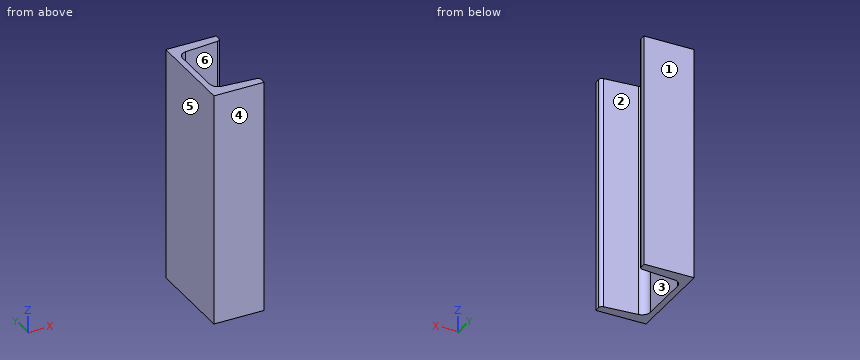
Autodesk Inventor part; units mm, degrees
ref_plane "Начальная плоскость" through (0, 0, 0) normal (0, 0, 1) x (1, 0, 0)
ref_plane "Конечная плоскость" through (0, 0, 168) normal (0, 0, 1) x (1, 0, 0)
ref_plane "YZ Plane" through (0, 0, 0) normal (1, 0, 0) x (0, 1, 0)
ref_plane "Начальная плоскость" through (0, 0, 0) normal (0, 0, 1) x (1, 0, 0)
ref_plane "Конечная плоскость" through (0, 0, 168) normal (0, 0, 1) x (1, 0, 0)
sketch "Эскиз" plane through (0, 0, 0) normal (0, 0, 1) x (1, 0, 0)
  line L0 (36, -32.5) -> (0, -32.5)
  line L1 (36, -32.5) -> (36, -28.696)
  line L2 (33.6994, -26.2039) -> (9.9215, -24.3017)
  line L3 (4.4, -18.3208) -> (4.4, 18.3208)
  line L4 (33.6994, 26.2039) -> (9.9215, 24.3017)
  line L5 (36, 28.696) -> (36, 32.5)
  line L6 (0, 32.5) -> (36, 32.5)
  line L7 (0, -32.5) -> (0, 32.5)
  arc A0 (4.4, -18.3208) -> (9.9215, -24.3017) centre (10.4, -18.3208) ccw
  arc A1 (9.9215, 24.3017) -> (4.4, 18.3208) centre (10.4, 18.3208) ccw
  arc A2 (36, -28.696) -> (33.6994, -26.2039) centre (33.5, -28.696) ccw
  arc A3 (33.6994, 26.2039) -> (36, 28.696) centre (33.5, 28.696) ccw
  line L8 (0, 45.5) -> (0, -45.5) construction
  line L9 (-7.2974, 0) -> (43.7847, 0) construction
  point P0 (36, -26.388)
  point P1 (4.4, -23.86)
  point P2 (4.4, 23.86)
  point P3 (36, 26.388)
  dimension "d3" = 36
  dimension "d5" = 4.4
  dimension "d7" = 65
  dimension "d9" = 8.64
  dimension "d11" = 8.64
  dimension "d13" = 6.112
  dimension "d15" = 6.112
  dimension "d22" = 6
  dimension "d23" = 2.5
  dimension "d24" = 32.5
  dimension "d25" = 0
extrude "Тело" add sketch "Эскиз" along normal up to surface (168 mm away) from surface at 0
sketch "Sketch3" plane through (0, 0, 0) normal (0, 0, 1) x (1, 0, 0)
  line L0 (0, 0) -> (10, 0)
ref_plane "Work Plane7" through (0, 0, 0) normal (0, -1, 0) x (1, 0, 0)
sketch "Sketch4" plane through (0, 0, 0) normal (0, -1, 0) x (1, 0, 0)
  line L0 (-2, 0) -> (12, 0)
  line L1 (-2, 168) -> (12, 168)
  dimension "d29" = 168
equation "\"d3\" = b"
equation "\"d7\" = ParH"
equation "\"d22\" = R"
equation "\"d23\" = R1"
equation "\"d24\" = 0.5 * d7"
equation "\"d16\" = G_L"
equation "\"R1\" = 2.5"
equation "\"R\" = 6"
equation "\"t1\" = 4.4"
equation "\"t2\" = 7.2"
equation "\"ParH\" = 65"
equation "\"b\" = 36"
equation "\"msp_x1\" = 0.04 * b"
equation "\"msp_x2\" = -0.08 * t1 + 0.04 * b"
equation "\"G_L\" = d29"
equation "\"ex\" = 0"
equation "\"G_OFFSET_START\" = 0"
equation "\"G_OFFSET_END\" = 0"
equation "\"d27\" = G_OFFSET_END + B_L"
equation "\"B_L\" = 168"
properties part number "Швеллер 6.5U-168 ГОСТ 8240-97" material "Сталь, мягкая"
Build history of the part. All positions in model axes, mm. Face numbers are marked on the shaded views. A direction names the side the tool comes from. Round coordinates to 2 decimals unless told otherwise and drop trailing zeros. Order: outer loops, then holes, each group sorted by start corner. A loop starts at its lowest first (then second) coordinate and runs counter-clockwise, first axis right, second up. Notation, with made-up numbers: (72.5, -10.75) - (98.5, -10.75) arc R15 ccw to (98.5, 10.25) - close; hole circle Ø5 at (-20, 10). An arc over 180 degrees is marked (long way). Use a Markdown table: item, result.
1) Pull direction Y, two halves, no side cores. Call the marked faces 3, 4, 5 and 6: pulls with the +Y half, pulls with the -Y half, needs draft (parallel to the pull), parting line crosses it, or undercut.
Recorded:
| item | result |
|---|---|
| face 3 | undercut |
| face 4 | pulls with the -Y half |
| face 5 | needs draft |
| face 6 | undercut |
2) Saw through at C-C on y = 2.5. Write the cut outline in (x, z).
Recorded:
| item | result |
|---|---|
| outline | (0, 0) - (4.4, 0) - (4.4, 168) - (0, 168) - close |
3) Flat gauge pins, fed straight in: pin 1 Ø10 at (x, y) = (32, -23) entering from -Z; pin 2 Ø6 at (y, z) = (0.5, 147.5) entering from +X. Where does each tip first touch, or does it go through?
Recorded:
| item | result |
|---|---|
| pin 1 | stops at z = 0 |
| pin 2 | stops at x = 4.4 |
4) Saw through at B-B on z = 127.5. Write the cut outline in (x, y), and give its area (3 significant figures).
Recorded:
| item | result |
|---|---|
| outline | (0, -32.5) - (36, -32.5) - (36, -28.7) arc R2.5 ccw to (33.7, -26.2) - (9.92, -24.3) arc R6 cw to (4.4, -18.32) - (4.4, 18.32) arc R6 cw to (9.92, 24.3) - (33.7, 26.2) arc R2.5 ccw to (36, 28.7) - (36, 32.5) - (0, 32.5) - close |
| area | 763 mm² |
5) Saw through at A-A on x = 13.5. Write the cut outline in (y, z).
Recorded:
| item | result |
|---|---|
| outline | (-32.5, 0) - (-24.59, 0) - (-24.59, 168) - (-32.5, 168) - close; (24.59, 0) - (32.5, 0) - (32.5, 168) - (24.59, 168) - close |
6) Saw through at D-D on x = 29.5. Write the cut outline in (y, z).
Recorded:
| item | result |
|---|---|
| outline | (-32.5, 0) - (-25.87, 0) - (-25.87, 168) - (-32.5, 168) - close; (25.87, 0) - (32.5, 0) - (32.5, 168) - (25.87, 168) - close |
7) Tool access for the marked faces 1 and 2: list every direction of +Z, -Z, +X, -X, +Y, -Y with a clear straight run to the whole face (end or side of a thin tool).
Recorded:
| item | result |
|---|---|
| face 1 | +Z, -Z, +X, -X, +Y |
| face 2 | +Z, -Z, +X |
8) Wall check: L1, parallel to Y at x = 10, z = 98.5; L2, parallel to X at y = -16.5, z = 30; L3, parallel to Y at x = 12, z = 104.5. Give the ranges that are in metal, low to high.
Recorded:
| item | result |
|---|---|
| L1 | y = -32.5 to -24.31, 24.31 to 32.5 |
| L2 | x = 0 to 4.4 |
| L3 | y = -32.5 to -24.47, 24.47 to 32.5 |
